Study the drawing (mm; zero at the part's minimum x, y, z) and answer. Give positions to 0.01 mm unless a question says otherwise; leave off trailing zeros. Order: outer loops, then holes, each group sorted by start corner. A loop starts at its lowest first (then second) coordinate and runs counter-clockwise, first axis right, second up.
Item 1: Given pin 1 Ø2.5 at (x, y) = (159.5, 13.5) entering from -Z; pin 2 Ø0.9 at (x, y) = (189.5, 8) entering from +Z; pin 3 Ø0.9 at (x, z) = (178.5, 8) entering from +Y; pin 4 Ø0.9 at (x, z) = (174, 7) entering from -Y, each flat-ended and moving along its own axis, determine where each tip first touches the part or whether it passes through.
Item 2: Find the intervals of material crossed by line 1 along Z through (x, y) = (165.5, 13.5); line 2 along Z through (x, y) = (147, 8.75), in increasing order.
Item 3: A cutting plane is placed at A-A (x = 323). Write down the section's boundary in (y, z), plus the area to 3 significant figures.
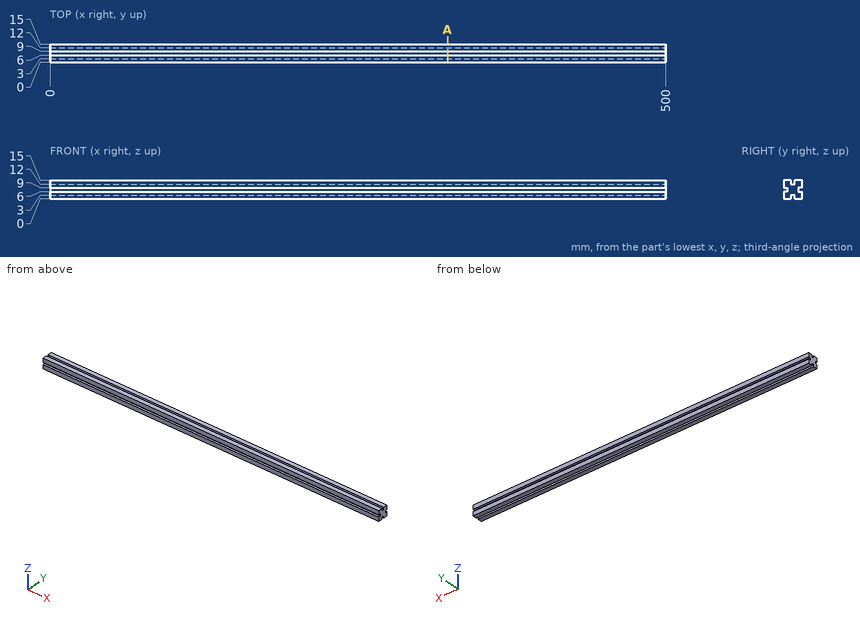
Response values:
1. pin 1: stops at z = 0
1. pin 2: stops at z = 12
1. pin 3: stops at y = 12
1. pin 4: stops at y = 3
2. line 1: z = 0 to 6, 9 to 15
2. line 2: z = 3 to 12
3. outline: (0, 0) - (6, 0) - (6, 3) - (9, 3) - (9, 0) - (15, 0) - (15, 6) - (12, 6) - (12, 9) - (15, 9) - (15, 15) - (9, 15) - (9, 12) - (6, 12) - (6, 15) - (0, 15) - (0, 9) - (3, 9) - (3, 6) - (0, 6) - close
3. area: 189 mm2
